Input: dimensioned drawing with shaded views. Units: mm. Origin: part minimum x, y, z. A direction names the side the tool comes from. Round coordinates to 2 decimals unless told otherwise and drop trailing zeros. Loops run counter-clockwise (first coordinate to the right, second up) from the corner with the lowest first, then second, coordinate; pieces in that order, holes last. Notation, with made-up numbers: M -38,-26.75 L -10,-26.75 A5 cw -10,-20.75 Z; hole C 79,-19 d7. An arc over 180 degrees is marked long. One line per item, written item: value.
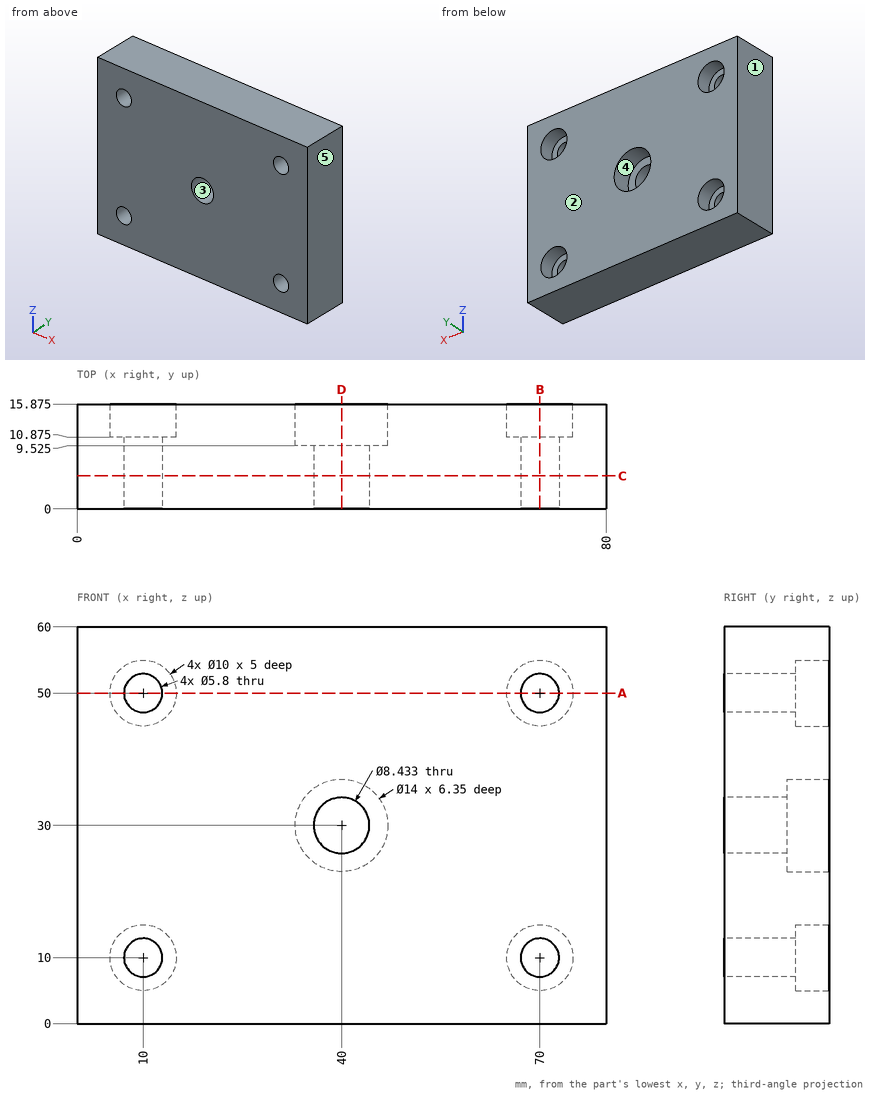
1. Section query D-D (x = 40). Return the cut outline in (y, z) (1 decimal), and give its area (3 significant figures).
Report:
outline: M 0,0 L 15.9,0 L 15.9,23 L 9.5,23 L 9.5,25.8 L 0,25.8 Z; M 0,34.2 L 9.5,34.2 L 9.5,37 L 15.9,37 L 15.9,60 L 0,60 Z
area: 783 mm2
2. Section query A-A (z = 50). Return the cut outline in (x, y) (3 decimals).
Report:
outline: M 0,0 L 7.1,0 L 7.1,10.875 L 5,10.875 L 5,15.875 L 0,15.875 Z; M 12.9,0 L 67.1,0 L 67.1,10.875 L 65,10.875 L 65,15.875 L 15,15.875 L 15,10.875 L 12.9,10.875 Z; M 72.9,0 L 80,0 L 80,15.875 L 75,15.875 L 75,10.875 L 72.9,10.875 Z
3. Pin query (flat end, axial travel): pin 1 (9 mm diameter, centred on x = 10, z = 10, fed in from -Y); pin 2 (6.5 mm diameter, centred on x = 70, z = 50, fed in from +Y) (3 decimals). Return the tip coordinate at first contact, or that it passes through.
Report:
pin 1: stops at y = 0
pin 2: stops at y = 10.875
4. Pull-direction query (X, two-part tool) for the marked faces 1, 2 and 3; classes: released by +X, released by -X, zero draft, split by the parting line, or undercut.
Report:
face 1: released by -X
face 2: zero draft
face 3: undercut
5. Reachability of the marked faces 4 and 5 from +Z, -Z, +X, -X, +Y, -Y: full face, straight path, thin tool, end or side. Return the list, or none.
Report:
face 4: +Y
face 5: +Z, -Z, +X, +Y, -Y
6. Section query B-B (x = 70). Return the cut outline in (y, z) (3 decimals).
Report:
outline: M 0,0 L 15.875,0 L 15.875,5 L 10.875,5 L 10.875,7.1 L 0,7.1 Z; M 0,12.9 L 10.875,12.9 L 10.875,15 L 15.875,15 L 15.875,45 L 10.875,45 L 10.875,47.1 L 0,47.1 Z; M 0,52.9 L 10.875,52.9 L 10.875,55 L 15.875,55 L 15.875,60 L 0,60 Z
7. Ray query, line 1 (X direction, y = 14.05, z = 50); line 2 (Z direction, x = 10, y = 14.9); line 3 (X direction, y = 3.25, z = 50). Return the intervals inside material, ascending. Write a range as [from, to].
Report:
line 1: x = [0, 5], [15, 65], [75, 80]
line 2: z = [0, 5], [15, 45], [55, 60]
line 3: x = [0, 7.1], [12.9, 67.1], [72.9, 80]
8. Section query C-C (y = 5). Return the cut outline in (x, z).
Report:
outline: M 0,0 L 80,0 L 80,60 L 0,60 Z; hole C 10,10 d5.8; hole C 10,50 d5.8; hole C 40,30 d8.43; hole C 70,10 d5.8; hole C 70,50 d5.8
